Autodesk Inventor part; units mm, degrees
ref_plane "YZ Plane" through (0, 0, 0) normal (1, 0, 0) x (0, 1, 0)
ref_plane "XZ Plane" through (0, 0, 0) normal (0, 1, 0) x (-1, 0, 0)
ref_plane "XY Plane" through (0, 0, 0) normal (0, 0, 1) x (1, 0, 0)
sketch "Sketch11" plane through (0, 0, 0) normal (0, 1, 0) x (-1, 0, 0)
  line L0 (0, 0) -> (16, 0)
  line L1 (16, 0) -> (16, -40)
  line L2 (16, -40) -> (0, -40)
  line L3 (0, -40) -> (0, 0)
  circle A0 centre (8, -24) radius 1
  circle A1 centre (4, -20) radius 1
  circle A2 centre (8, -16) radius 1
  circle A3 centre (12, -20) radius 1
  dimension "d45" = 16
  dimension "d46" = 40
  dimension "d47" = 2
  dimension "d48" = 2
  dimension "d49" = 2
  dimension "d50" = 2
  dimension "d51" = 8
  dimension "d52" = 24
  dimension "d53" = 8
  dimension "d54" = 24
  dimension "d55" = 12
  dimension "d56" = 20
  dimension "d57" = 20
  dimension "d58" = 4
extrude "Extrusion6" add sketch "Sketch11" along normal blind 3
sketch "Sketch12" plane through (0, 3, 0) normal (0, 1, 0) x (1, 0, 0)
  line L0 (-16, 40) -> (-16, 0)
  line L1 (0, 0) -> (-16, 0)
  line L2 (-16, 0) -> (-16, 3)
  line L3 (-16, 3) -> (0, 3)
  line L4 (0, 3) -> (0, 0)
  line L5 (0, 40) -> (-16, 40)
  line L6 (-16, 40) -> (-16, 37)
  line L7 (-16, 37) -> (0, 37)
  line L8 (0, 37) -> (0, 40)
  dimension "d61" = 3
  dimension "d62" = 3
extrude "Extrusion7" add sketch "Sketch12" along normal blind 25
fillet "Fillet3" radius 8 4 edges at (0, 28, -1.5) (-16, 28, -1.5) (-16, 28, -38.5) (0, 28, -38.5)
sketch "Sketch13" plane through (-16, 0, 0) normal (0, 0, 1) x (1, 0, 0)
  circle A0 centre (8, 20) radius 1
  circle A1 centre (8, 16) radius 0.5
  line L0 (16, 0) -> (0, 0)
  line L1 (16, 0) -> (16, 20)
  circle A2 centre (8, 12) radius 0.5
  circle A3 centre (8, 24) radius 0.5
  circle A4 centre (12, 20) radius 0.5
  circle A5 centre (4, 20) radius 0.5
  circle A6 centre (8, 8) radius 0.5
  dimension "d66" = 2
  dimension "d67" = 1
  dimension "d68" = 20
  dimension "d69" = 8
  dimension "d70" = 8
  dimension "d71" = 16
  dimension "d72" = 1
  dimension "d73" = 1
  dimension "d74" = 1
  dimension "d75" = 1
  dimension "d76" = 1
  dimension "d77" = 4
  dimension "d78" = 8
  dimension "d79" = 4
  dimension "d80" = 20
  dimension "d81" = 4
  dimension "d82" = 20
  dimension "d83" = 8
  dimension "d84" = 8
  dimension "d85" = 8
  dimension "d86" = 12
sketch "Sketch14" plane through (0, 0, -40) normal (0, 0, -1) x (-1, 0, 0)
  circle A0 centre (8, 20) radius 1
  circle A1 centre (8, 16) radius 0.5
  circle A2 centre (8, 12) radius 0.5
  circle A3 centre (12, 20) radius 0.5
  circle A4 centre (8, 24) radius 0.5
  circle A5 centre (4, 20) radius 0.5
  circle A6 centre (8, 8) radius 0.5
  line L0 (16, 0) -> (16, 20)
  line L1 (16, 0) -> (0, 0)
  line L2 (0, 0) -> (0, 20)
  dimension "d87" = 2
  dimension "d88" = 1
  dimension "d89" = 1
  dimension "d90" = 1
  dimension "d91" = 1
  dimension "d92" = 1
  dimension "d93" = 1
  dimension "d94" = 8
  dimension "d95" = 20
  dimension "d96" = 20
  dimension "d97" = 4
  dimension "d98" = 4
  dimension "d99" = 8
  dimension "d100" = 4
  dimension "d101" = 20
  dimension "d102" = 4
  dimension "d103" = 8
  dimension "d104" = 8
  dimension "d105" = 8
  dimension "d106" = 12
  dimension "d107" = 8
extrude "Extrusion8" cut sketch "Sketch14" against normal blind 3
extrude "Extrusion9" cut sketch "Sketch13" against normal blind 3
fillet "Fillet4" radius 0.5 18 edges at (-16, 11.5003, -3) (0, 11.5003, -3) (-2.343, 25.657, -3) (0, 10.0003, 0) (-16, 10.0003, 0) (-2.343, 25.657, 0) (0, 3, -20) (0, 0, -20) (-16, 3, -20) (-13.657, 25.657, -37) (-16, 11.5003, -37) (0, 11.5003, -37) (-13.657, 25.657, -40) (-16, 10.0003, -40) (0, 10.0003, -40) (-8, 0, 0) (-16, 0, -20) (-8, 0, -40)
equation "\"d51\" = 0.5 * d45"
equation "\"d53\" = 0.5 * d45"
equation "\"d56\" = 0.5 * d46"
equation "\"d57\" = 0.5 * d46"
properties part number "fork"
The model under review builds one solid part; all positions refer to its coordinate system, in mm. A direction names the side the tool comes from. Coordinates: 2 decimals unless noted, no trailing zeros. Write each loop counter-clockwise with the first axis right and the second up, starting at its lowest first coordinate (ties: lowest second). Pieces come first, ordered by that corner, then holes. Notation, with made-up numbers: (46, 41) - (68, 41) arc R24 cw to (68, 60) - close; hole circle Ø4 at (56.5, 53). An arc over 180 degrees is marked (long way). Answer in a Markdown table with one row per item. Add a question column.
Q1. Consider section D-D on z = -7.5. Give the boundary of the cut face in (x, y).
Q2. For faces 1 (the face through (-8, 15, -37)), 2 (the face through (-8, 14, 0)), list the 3-axis set-ups (+Z, -Z, +X, -X, +Y, -Y) from which the entire face can be reached by the end or side of a thin tool; tool diameter is ignored.
Q3. Consider section B-B on z = -16. Give the boundary of the cut face in (x, y), then the cut area to 3 significant figures.
Q4. To check wall thickness, follow line 1 along Y through (x, z) = (-8, -1); line 2 along Z through (x, y) = (-12.5, 5.75); line 3 along Y through (x, z) = (-2.25, -21). State the ranges of each line that lie inside material, in increasing order. Write a range as from..to.
Q5. Draft analysis for pull direction Y (two halves, no side actions). For faces 3 (the face through (-8, 0, -20)), 4 (the face through (-4.065, 20.496, -1.479)), 5 (the face through (-8.231, 7.556, -38.521)), 6 (the face through (-16, 2, -20)), state which applies: +Y half, -Y half, draft (parallel to the pull), parting line (faces both ways), or undercut.
Q6. Clearance check with flat-ended pins moving along their axes: pin 1 (8 mm diameter, centred on x = -8, y = 18.5, fed in from +Z); pin 2 (1.8 mm diameter, centred on x = -8, z = -16, fed in from +Y); pin 3 (3 mm diameter, centred on x = -8, z = -24, fed in from +Y). State where each tip first meets the part, or that it passes through.
Q7. Consider section C-C on z = -20. Give the boundary of the cut face in (x, y).
Q8. Consider section A-A on y = 8. Give the boundary of the cut face in (x, z).
Answers below:
| question | item | result |
|---|---|---|
| 1 | outline | (-16, 0.5) arc R0.5 ccw to (-15.5, 0) - (-0.5, 0) arc R0.5 ccw to (0, 0.5) - (0, 2.5) arc R0.5 ccw to (-0.5, 3) - (-15.5, 3) arc R0.5 ccw to (-16, 2.5) - close |
| 2 | face 1 | +X, -X, +Y |
| 2 | face 2 | +Z, +X, -X, +Y, -Y |
| 3 | outline | (-16, 0.5) arc R0.5 ccw to (-15.5, 0) - (-9, 0) - (-9, 3) - (-15.5, 3) arc R0.5 ccw to (-16, 2.5) - close; (-7, 0) - (-0.5, 0) arc R0.5 ccw to (0, 0.5) - (0, 2.5) arc R0.5 ccw to (-0.5, 3) - (-7, 3) - close |
| 3 | area | 41.8 mm² |
| 4 | line 1 | 0..7.5, 8.5..11.5, 12.5..15.5, 16.5..19, 21..23.5, 24.5..28 |
| 4 | line 2 | -40..-37, -3..0 |
| 4 | line 3 | 0..3 |
| 5 | face 3 | -Y half |
| 5 | face 4 | undercut |
| 5 | face 5 | undercut |
| 5 | face 6 | draft |
| 6 | pin 1 | z = 0 |
| 6 | pin 2 | through |
| 6 | pin 3 | y = 3 |
| 7 | outline | (-16, 0.5) arc R0.5 ccw to (-15.5, 0) - (-13, 0) - (-13, 3) - (-15.5, 3) arc R0.5 ccw to (-16, 2.5) - close; (-11, 0) - (-5, 0) - (-5, 3) - (-11, 3) - close; (-3, 0) - (-0.5, 0) arc R0.5 ccw to (0, 0.5) - (0, 2.5) arc R0.5 ccw to (-0.5, 3) - (-3, 3) - close |
| 8 | outline | (-16, -39.5) arc R0.5 ccw to (-15.5, -40) - (-8.5, -40) - (-8.5, -37) - (-15.5, -37) arc R0.5 ccw to (-16, -37.5) - close; (-16, -2.5) arc R0.5 ccw to (-15.5, -3) - (-8.5, -3) - (-8.5, 0) - (-15.5, 0) arc R0.5 ccw to (-16, -0.5) - close; (-7.5, -40) - (-0.5, -40) arc R0.5 ccw to (0, -39.5) - (0, -37.5) arc R0.5 ccw to (-0.5, -37) - (-7.5, -37) - close; (-7.5, -3) - (-0.5, -3) arc R0.5 ccw to (0, -2.5) - (0, -0.5) arc R0.5 ccw to (-0.5, 0) - (-7.5, 0) - close |
